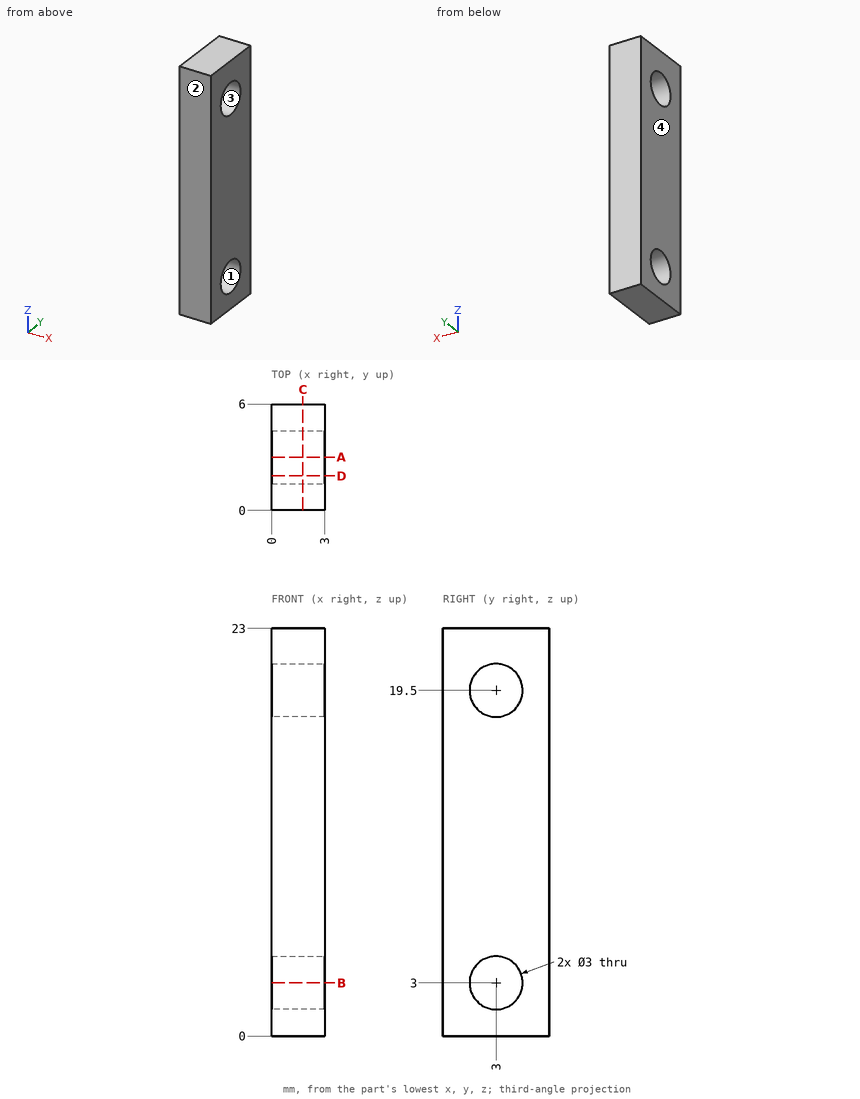
Design review of the part shown in the three views and the two pictorial views. Dimensions are in mm from the part's minimum x, y and z. Round coordinates to 2 decimals unless told otherwise and drop trailing zeros. Write each loop counter-clockwise with the first axis right and the second up, starting at its lowest first coordinate (ties: lowest second). Pieces come first, ordered by that corner, then holes. Notation, with made-up numbers: (56, -17) -> (71, -17) arc R17 ccw to (71, -9) -> close; hole circle Ø11 at (44, 31). An arc over 180 degrees is marked (long way). Answer as a JSON object with one key per item and string values.
1. We need section C-C on x = 1.75. State the section outline as (y, z) points, and give its area (3 significant figures).
Results found:
{"outline": "(0, 0) -> (6, 0) -> (6, 23) -> (0, 23) -> close; hole circle Ø3 at (3, 3); hole circle Ø3 at (3, 19.5)", "area": "124 mm^2"}
2. We need section D-D on y = 1.95. State the section outline as (x, z) points, and give its area (3 significant figures).
Results found:
{"outline": "(0, 0) -> (3, 0) -> (3, 1.93) -> (0, 1.93) -> close; (0, 4.07) -> (3, 4.07) -> (3, 18.43) -> (0, 18.43) -> close; (0, 20.57) -> (3, 20.57) -> (3, 23) -> (0, 23) -> close", "area": "56.1 mm^2"}
3. We need section B-B on z = 3. State the section outline as (x, y) points.
Results found:
{"outline": "(0, 0) -> (3, 0) -> (3, 1.5) -> (0, 1.5) -> close; (0, 4.5) -> (3, 4.5) -> (3, 6) -> (0, 6) -> close"}
4. To check wall thickness, follow line 1 along Z through (x, y) = (1.3, 2.8); line 2 along Z through (x, y) = (1.4, 4.15); line 3 along Y through (x, z) = (1.55, 3). State the ranges of each line that lie inside material, in increasing order.
Results found:
{"line 1": "z = 0 to 1.51, 4.49 to 18.01, 20.99 to 23", "line 2": "z = 0 to 2.04, 3.96 to 18.54, 20.46 to 23", "line 3": "y = 0 to 1.5, 4.5 to 6"}
5. The part is to be moulded in two halves that separate along Y. For the marked faces 1, 2, 3 and 4, say which applies: pulls with the +Y half, pulls with the -Y half, needs draft (parallel to the pull), parting line crosses it, or undercut.
Results found:
{"face 1": "undercut", "face 2": "pulls with the -Y half", "face 3": "undercut", "face 4": "needs draft"}
6. We need section A-A on y = 3. State the section outline as (x, z) points.
Results found:
{"outline": "(0, 0) -> (3, 0) -> (3, 1.5) -> (0, 1.5) -> close; (0, 4.5) -> (3, 4.5) -> (3, 18) -> (0, 18) -> close; (0, 21) -> (3, 21) -> (3, 23) -> (0, 23) -> close"}
